The listing builds one solid part. Answer for the finished solid, in the listing's coordinates (mm). A direction names the side the tool comes from. Coordinates: 2 decimals unless noted, no trailing zeros. Order: outer loops, then holes, each group sorted by start corner. A loop starts at its lowest first (then second) coordinate and runs counter-clockwise, first axis right, second up. Notation, with made-up numbers: (89, -26.75) -> (130, -26.75) arc R19 cw to (130, -10.75) -> close; hole circle Ø11 at (-23, 75). An arc over 180 degrees is marked (long way). Put each result on its own line as item: value. Start each with the question number.
```python
from build123d import *

# Parameters (mm, degrees)
SKETCH2_W           = 25.8
SKETCH2_H           = 49.8
BOSS_EXTRUDE1_DEPTH = 13.1
SKETCH3_R           = 5
BOSS_EXTRUDE2_DEPTH = 105.5


with BuildPart() as part:
    # Sketch2 → Boss-Extrude1 (new body)
    with BuildSketch(Plane.XY):
        with Locations((12.9, 24.9)):
            Rectangle(SKETCH2_W, SKETCH2_H)
    extrude(amount=BOSS_EXTRUDE1_DEPTH)

    # Sketch3 → Boss-Extrude2 (add)
    with BuildSketch(Plane(origin=(0, 49.8, 0), x_dir=(1, 0, 0), z_dir=(0, 1, 0))):
        with Locations((20.8, -6.55)):
            Circle(SKETCH3_R)
    extrude(amount=BOSS_EXTRUDE2_DEPTH)


solid = part.part
```
(1) The part is cut by section B-B on x = 17.25. Determine the outline of the cut face in (y, z).
(2) The part is cut by section C-C on y = 75. Determine the outline of the cut face in (x, z).
(3) A tool of negligible diameter and unlimited length cuts with its end or side. For faces 1 (the cylindrical face through (16.83, 101.81, 9.59)), 2 (the flat face through (0, 25, 6)), from which of +Z, -Z, +X, -X, +Y, -Y can it reach the whole face along a straight path? Write none if from no direction.
(4) The part is cut by section A-A on z = 3.5. Determine the outline of the cut face in (x, y).
(5) Find the intervals of material crossed by L1, parallel to Y at x = 4.25, z = 1.75; L2, parallel to X at y = 66, z = 10.5; L3, parallel to Z at x = 17.5, y = 115, in increasing order.
(6) Each of these flat-tipped pins is pushed along its axis until it touches: P1, Ø10, axis at x = 15, y = 65.5, coming from the +Z side; P2, Ø3, axis at x = 13, z = 7, coming from the +Y side; P3, Ø3, axis at x = 15.5, z = 3.5, coming from the -Y side; P4, Ø5, axis at x = 22, y = 122.5, coming from the -Z side. Where does it stop, or does it pass through?
Worked out:
1. outline: (0, 0) -> (49.8, 0) -> (49.8, 3.03) -> (155.3, 3.03) -> (155.3, 10.07) -> (49.8, 10.07) -> (49.8, 13.1) -> (0, 13.1) -> close
2. outline: circle Ø10 at (20.8, 6.55)
3. face 1: +Y
3. face 2: +Z, -Z, -X, +Y, -Y
4. outline: (0, 0) -> (25.8, 0) -> (25.8, 49.8) -> (24.76, 49.8) -> (24.76, 155.3) -> (16.84, 155.3) -> (16.84, 49.8) -> (0, 49.8) -> close
5. L1: 0 to 49.8
5. L2: 17.73 to 23.87
5. L3: 2.79 to 10.31
6. P1: z = 11.49
6. P2: y = 49.8
6. P3: y = 0
6. P4: z = 1.55
